Autodesk Inventor part; units mm, degrees
ref_plane "YZ Plane" through (0, 0, 0) normal (1, 0, 0) x (0, 1, 0)
ref_plane "XZ Plane" through (0, 0, 0) normal (0, 1, 0) x (-1, 0, 0)
ref_plane "XY Plane" through (0, 0, 0) normal (0, 0, 1) x (1, 0, 0)
sketch "Эскиз1" plane through (0, 0, 0) normal (0, 1, 0) x (-1, 0, 0)
  line L0 (45, 15) -> (-45, 15)
  line L1 (-45, 15) -> (-45, -15)
  line L2 (-45, -15) -> (45, -15)
  line L3 (45, -15) -> (45, 15)
  line L4 (45, 15) -> (-45, -15) construction
  line L5 (-45, 15) -> (45, -15) construction
  line L6 (-45, 15) -> (-9, 15)
  line L7 (-9, 15) -> (-9, 0)
  line L8 (-9, 0) -> (13, 0)
  line L9 (13, 0) -> (-9, 0) construction
  line L10 (-45, -15) -> (-34, -15)
  line L11 (-34, -15) -> (-34, 0)
  line L12 (-34, 0) -> (-34, -6)
  line L13 (-45, -15) -> (-45, -14)
  line L14 (-45, 15) -> (-45, 14)
  line L15 (-45, -14) -> (-28.0294, -14) construction
  line L16 (-34, -6) -> (-37, -6)
  line L17 (-34, 0) -> (-34, 6)
  line L18 (-34, 6) -> (-37, 6)
  line L19 (-37, 6) -> (-45, 14)
  line L20 (-45, -14) -> (-37, -6)
  line L21 (-45, 0) -> (-51.506, 0)
  circle A0 centre (-51, 0) radius 14.1421
  line L22 (-9, 0) -> (13, 0) construction
  line L23 (-9, -4) -> (13, -4)
  line L24 (13, 4) -> (-9, 4)
  arc A1 (-9, 4) -> (-9, -4) centre (-9, 0) ccw
  arc A2 (13, -4) -> (13, 4) centre (13, 0) ccw
  point P0 (0, 0)
  point P1 (2, 0)
  point P2 (2, 0)
  dimension "d0" = 90
  dimension "d1" = 30
  dimension "d2" = 36
  dimension "d3" = 22
  dimension "d7" = 11
  dimension "d8" = 6
  dimension "d9" = 1
  dimension "d10" = 1
  dimension "d12" = 6
  dimension "d13" = 3
  dimension "d14" = 6.506
  dimension "d17" = 8
extrude "Выдавливание1" add sketch "Эскиз1" along normal blind 39 contours L3 L2 L11 L17 L18 L19 L1 L0 | L2 L1 L20 L16 L11 | A1 L24 A2 L23
extrude "Выдавливание2" cut sketch "Эскиз1" along normal blind 2 contours A1 L24 A2 L23
mirror "Зеркальное отражение1" about plane through (0, 39, 0) normal (0, 1, 0) of "Выдавливание2", "Выдавливание1"
chamfer "Фаска1" distance 2 angle 45 2 edges at (-45, 39, -15) (-45, 39, 15)
properties part number "Призма-5"
Input: part model. Units: mm. Frame: model coordinates. A direction names the side the tool comes from. Coordinates: 2 decimals unless noted, no trailing zeros. Loops run counter-clockwise (first coordinate to the right, second up) from the corner with the lowest first, then second, coordinate; pieces in that order, holes last.
Q1. Mould query, pull axis Z, two halves, no side actions, for faces 1 (the flat face through (-45, 38, 0)), 2 (the flat face through (-2, 77, 4)), 3 (the flat face through (0, 38, 15)). Classes: +Z half, -Z half, draft (parallel to the pull), parting line (faces both ways), or undercut.
Results are:
face 1: draft
face 2: undercut
face 3: +Z half
Q2. Set-up query: faces 4 (the flat face through (-2, 76, 0)), 5 (the flat face through (-2, 2, 0)), 6 (the flat face through (41, 38, -10)). Return all of +Z, -Z, +X, -X, +Y, -Y with unobstructed straight access to the full face (end or side cutting, diameter ignored); none if empty.
Results are:
face 4: +Y
face 5: -Y
face 6: +X, +Y, -Y
Q3. Section A-A, the plane z = 0. Return the cut outline in (x, y), and give its area (3 significant figures).
Results are:
outline: (-45, 0) - (-17, 0) - (-17, 2) - (13, 2) - (13, 0) - (34, 0) - (34, 78) - (13, 78) - (13, 76) - (-17, 76) - (-17, 78) - (-45, 78) - close
area: 6,040 mm2
Q4. Section B-B, the plane y = 20.5. Return the cut outline in (x, z), and give its area (3 significant figures).
Results are:
outline: (-45, -13) - (-43, -15) - (45, -15) - (45, -14) - (37, -6) - (34, -6) - (34, 6) - (37, 6) - (45, 14) - (45, 15) - (-43, 15) - (-45, 13) - close
area: 2,500 mm2
Q5. Line query: line 1 along Y through (x, z) = (11.5, 0.25); line 2 along Z through (x, y) = (39.5, 31.5); line 3 along X through (y, z) = (40.5, 3.5). Output: solid intervals per line, ascending.
Results are:
line 1: y = 2 to 76
line 2: z = -15 to -8.5, 8.5 to 15
line 3: x = -45 to 34
Q6. Contact query for flat-ended pins moving along their axis: pin 1 (9.5 mm diameter, centred on y = 37, z = 0, fed in from +X); pin 2 (6.5 mm diameter, centred on x = -8.5, z = -2, fed in from +Y); pin 3 (6 mm diameter, centred on y = 53, z = 7, fed in from +X); pin 4 (8 mm diameter, centred on y = 10.5, z = 2.5, fed in from +X). Output: stop coordinate, or through.
Results are:
pin 1: stops at x = 34
pin 2: stops at y = 78
pin 3: stops at x = 41
pin 4: stops at x = 37.5
